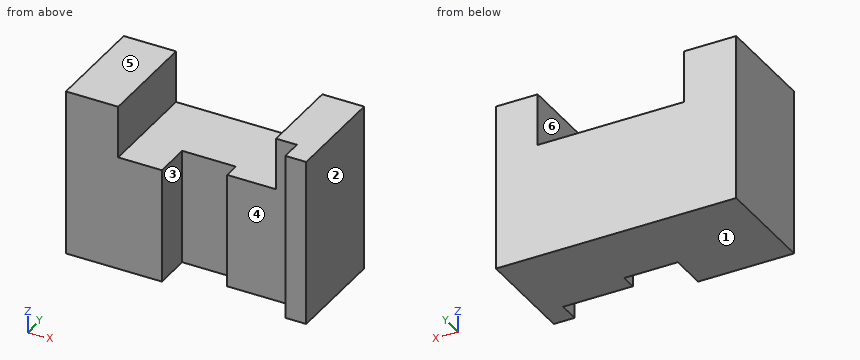
```python
from build123d import *

# Parameters (mm, degrees)
F1_DEPTH = 50
F2_W     = 25.703896
F2_H     = 55
F3_DEPTH = 17.5
F4_DEPTH = 10


with BuildPart() as f1:
    # F0 (on Front) → F1 (new body)
    with BuildSketch(Plane.XZ):
        Polygon((25, 80), (0, 80), (0, 0), (115, 0), (115, 80), (95, 80), (95, 55), (25, 55), align=None)
    extrude(amount=F1_DEPTH)

    # F2 (on face) → F3 (cut, symmetric)
    with BuildSketch(Plane.XZ.offset(50)):
        with Locations((58.791665, 27.5)):
            Rectangle(F2_W, F2_H)
    extrude(amount=F3_DEPTH, both=True, mode=Mode.SUBTRACT)

    # F2 (on face) → F4 (cut)
    with BuildSketch(Plane.XZ.offset(50)):
        Polygon((95, 55), (71.643613, 55), (71.643613, 0), (105, 0), (105, 80), (95, 80), align=None)
    extrude(amount=-F4_DEPTH, mode=Mode.SUBTRACT)


solid = f1.part
```
Work out the finished part from the listing and answer in its coordinate system (mm). Face numbers are marked on the shaded views. A direction names the side the tool comes from. Give positions to 0.01 mm unless a question says otherwise; leave off trailing zeros. Order: outer loops, then holes, each group sorted by start corner. A loop starts at its lowest first (then second) coordinate and runs counter-clockwise, first axis right, second up.
1. Section B-B, the plane z = 36 is taken. Determine the outline of the cut face in (x, y), and give its area (3 significant figures).
Result sheet:
outline: (0, -50) - (45.94, -50) - (45.94, -32.5) - (71.64, -32.5) - (71.64, -40) - (105, -40) - (105, -50) - (115, -50) - (115, 0) - (0, 0) - close
area: 4,970 mm2
2. The mould has two halves that part along X. Classify the marked faces 1, 2 and 3: released by +X, released by -X, zero draft, split by the parting line, or undercut.
Result sheet:
face 1: zero draft
face 2: released by +X
face 3: undercut
3. For the marked faces 4, 5 and 6, determine the directions among +Z, -Z, +X, -X, +Y, -Y from which every point of the face is accessible in a straight line to the end or side of a thin tool.
Result sheet:
face 4: +Z, -Z, -Y
face 5: +Z, +X, -X, +Y, -Y
face 6: +Z, +Y, -Y
4. Straight lines are drawn through the part: L1, parallel to X at y = -24, z = 73.5; L2, parallel to X at y = -46, z = 31.5; L3, parallel to Z at x = 35.5, y = -42. For each, find the intervals that lie inside material, in ascending order.
Result sheet:
L1: x = 0 to 25, 95 to 115
L2: x = 0 to 45.94, 105 to 115
L3: z = 0 to 55
5. Each of these flat-tipped pins is pushed along its axis until it touches: P1, Ø1.5, axis at x = 51.5, z = 41, coming from the -Y side; P2, Ø5, axis at x = 92.5, z = 21, coming from the -Y side. Where does it stop, or does it pass through?
Result sheet:
P1: stops at y = -32.5
P2: stops at y = -40
6. Section C-C, the plane y = -20 is taken. Determine the outline of the cut face in (x, z).
Result sheet:
outline: (0, 0) - (115, 0) - (115, 80) - (95, 80) - (95, 55) - (25, 55) - (25, 80) - (0, 80) - close
7. Section A-A, the plane y = -43 is taken. Determine the outline of the cut face in (x, z).
Result sheet:
outline: (0, 0) - (45.94, 0) - (45.94, 55) - (25, 55) - (25, 80) - (0, 80) - close; (105, 0) - (115, 0) - (115, 80) - (105, 80) - close
8. Section D-D, the plane x = 29.5 is taken. Determine the outline of the cut face in (y, z).
Result sheet:
outline: (-50, 0) - (0, 0) - (0, 55) - (-50, 55) - close
